Geometry check sheet. Reference: the model listing, model coordinates, mm. A direction names the side the tool comes from. Round coordinates to 2 decimals unless told otherwise and drop trailing zeros. Loops run counter-clockwise (first coordinate to the right, second up) from the corner with the lowest first, then second, coordinate; pieces in that order, holes last. Notation, with made-up numbers: M -25,-30.75 L 30,-30.75 A22 cw 30,-5.75 Z; hole C 43,-22 d6. An arc over 180 degrees is marked long. Answer in a Markdown table with one row per item. Add a question column.
```python
from build123d import *

# Parameters (mm, degrees)
BOSS_EXTRUDE1_DEPTH = 50
SKETCH2_R           = 7.75
CUT_EXTRUDE1_DEPTH  = 12.25
SKETCH4_R           = 12
CUT_EXTRUDE2_DEPTH  = 5
SKETCH5_W           = 10
SKETCH5_H           = 14
CUT_EXTRUDE3_DEPTH  = 8
SKETCH6_R           = 2.1
CUT_EXTRUDE4_DEPTH  = 7
SKETCH7_W           = 14
SKETCH7_H           = 14.5
BOSS_EXTRUDE2_DEPTH = 9.77


with BuildPart() as part:
    # Sketch1 → Boss-Extrude1 (new body)
    with BuildSketch(Plane.XY):
        with BuildLine():
            Line((-7, 30), (7, 30))
            Line((7, 30), (7, 16.75))
            ThreePointArc((7, 16.75), (2.75, 12.5), (7, 8.25))
            Line((7, 8.25), (7, -8.25))
            ThreePointArc((7, -8.25), (2.75, -12.5), (7, -16.75))
            Line((7, -16.75), (7, -30))
            Line((7, -30), (-7, -30))
            Line((-7, -30), (-7, 30))
        make_face()
    extrude(amount=BOSS_EXTRUDE1_DEPTH)

    # Sketch2 → Cut-Extrude1 (cut, symmetric)
    with BuildSketch(Plane(origin=(0, 0, 25), x_dir=(-1, 0, 0), z_dir=(0, 0, -1))):
        with Locations((-7, 12.5)):
            Circle(SKETCH2_R)
    extrude(amount=CUT_EXTRUDE1_DEPTH, both=True, mode=Mode.SUBTRACT)

    # Sketch4 → Cut-Extrude2 (cut)
    with BuildSketch(Plane(origin=(0, 0, 23), x_dir=(-1, 0, 0), z_dir=(0, 0, -1))):
        with Locations((-7, -12.5)):
            Circle(SKETCH4_R)
    cut_extrude2 = extrude(amount=CUT_EXTRUDE2_DEPTH, mode=Mode.SUBTRACT)

    # Mirror1: Cut-Extrude2 across plane
    add(cut_extrude2.mirror(Plane(origin=(0, 0, 25), x_dir=(1, 0, 0), z_dir=(0, 0, -1))), mode=Mode.SUBTRACT)

    # Sketch5 → Cut-Extrude3 (cut)
    with BuildSketch(Plane.ZY.offset(7)):
        with Locations((5, 23)):
            Rectangle(SKETCH5_W, SKETCH5_H)
        with Locations((45, 23)):
            Rectangle(SKETCH5_W, SKETCH5_H)
        with Locations((45, -23)):
            Rectangle(SKETCH5_W, SKETCH5_H)
        with Locations((5, -23)):
            Rectangle(SKETCH5_W, SKETCH5_H)
    extrude(amount=-CUT_EXTRUDE3_DEPTH, mode=Mode.SUBTRACT)

    # Sketch6 → Cut-Extrude4 (cut, through all)
    with BuildSketch(Plane.ZY.offset(-1)):
        with Locations((5, 23)):
            Circle(SKETCH6_R)
        with Locations((45, 23)):
            Circle(SKETCH6_R)
        with Locations((5, -23)):
            Circle(SKETCH6_R)
        with Locations((45, -23)):
            Circle(SKETCH6_R)
    extrude(amount=-CUT_EXTRUDE4_DEPTH, mode=Mode.SUBTRACT)

    # Sketch7 → Boss-Extrude2 (add)
    with BuildSketch(Plane(origin=(0, 30, 0), x_dir=(1, 0, 0), z_dir=(0, 1, 0))):
        with Locations((0, -25)):
            Rectangle(SKETCH7_W, SKETCH7_H)
    extrude(amount=BOSS_EXTRUDE2_DEPTH)


solid = part.part
```
1) Thickness scan on L1, parallel to Z at x = -1.75, y = -8; L2, parallel to Z at x = 0.5, y = 11.5; L3, parallel to Y at x = -5.5, z = 10.5. Record the ranges inside material, lowest first. Write a range as [from, to].
2) Cross-section at B-B, the plane y = 23. Record the boundary of the cut face in (x, z).
3) Cross-section at A-A, the plane z = 5. Record the boundary of the cut face in (x, y).
4) Set-up check for faces 1 (the flat face through (-3, -23, 40)), 2 (the flat face through (1, -12, 18)), 3 (the flat face through (-3, -16, 5)), 4 (the flat face through (-3, 16, 45)): record each of +Z, -Z, +X, -X, +Y, -Y from which the full face is reachable in a straight line by a thin tool's end or side.
5) Cross-section at C-C, the plane z = 11.5. Record the boundary of the cut face in (x, y).
6) Cross-section at D-D, the plane x = 4. Count the separate pieces of the cut face and the enclosed holes in it, plus the area to 3 significant figures.
7) Go/stop test with flat-tipped pins: pin 1 (6 mm diameter, centred on x = -1, y = -13, fed in from -Z); pin 2 (4 mm diameter, centred on y = -23, z = 5, fed in from +X) (1 decimal); pin 3 (3 mm diameter, centred on y = 25.5, z = 4, fed in from -X); pin 4 (4 mm diameter, centred on x = 0, z = 43.5, fed in from +Y). Record where each tip stops, or that it passes through.
8) Draft check along Z on faces 5 (the flat face through (2, 13, 12.75)), 6 (the flat face through (0, 0, 50)), 7 (the flat face through (1, 23.1, 2.7)). Enter one of: +Z half, -Z half, draft (parallel to the pull), parting line (faces both ways), or undercut.
Worked answers:
| question | item | result |
|---|---|---|
| 1 | L1 | z = [0, 18], [23, 27], [32, 50] |
| 1 | L2 | z = [0, 12.75], [37.25, 50] |
| 1 | L3 | y = [-30, 30] |
| 2 | outline | M -7,10 L 1,10 L 1,7.1 L 7,7.1 L 7,42.9 L 1,42.9 L 1,40 L -7,40 Z; M 1,0 L 7,0 L 7,2.9 L 1,2.9 Z; M 1,47.1 L 7,47.1 L 7,50 L 1,50 Z |
| 3 | outline | M -7,-16 L 1,-16 L 1,-20.9 L 7,-20.9 L 7,-16.75 A4.25 cw 7,-8.25 L 7,8.25 A4.25 cw 7,16.75 L 7,20.9 L 1,20.9 L 1,16 L -7,16 Z; M 1,-30 L 7,-30 L 7,-25.1 L 1,-25.1 Z; M 1,25.1 L 7,25.1 L 7,30 L 1,30 Z |
| 4 | face 1 | +Z, -X, -Y |
| 4 | face 2 | +X |
| 4 | face 3 | -Z, -X, -Y |
| 4 | face 4 | +Z, -X, +Y |
| 5 | outline | M -7,-30 L 7,-30 L 7,-16.75 A4.25 cw 7,-8.25 L 7,8.25 A4.25 cw 7,16.75 L 7,30 L -7,30 Z |
| 6 | separate pieces | 3 |
| 6 | enclosed holes | 4 |
| 6 | area | 2,110 mm2 |
| 7 | pin 1 | stops at z = 0 |
| 7 | pin 2 | passes through |
| 7 | pin 3 | stops at x = 1 |
| 7 | pin 4 | stops at y = 30 |
| 8 | face 5 | undercut |
| 8 | face 6 | +Z half |
| 8 | face 7 | draft |
